For this review, take the finished solid that the model builds, in its own axes (mm). A direction names the side the tool comes from. Coordinates: 2 decimals unless noted, no trailing zeros. Loops run counter-clockwise (first coordinate to the right, second up) from the corner with the lowest first, then second, coordinate; pieces in that order, holes last.
```python
from build123d import *

# Parameters (mm, degrees)
SKETCH1_W           = 50
SKETCH1_H           = 60
BOSS_EXTRUDE1_DEPTH = 50
SKETCH2_W           = 30
SKETCH2_H           = 50
CUT_EXTRUDE1_DEPTH  = 77.811457479
SKETCH3_R           = 1.7
CUT_EXTRUDE2_DEPTH  = 64.442887702
SKETCH4_R           = 1.7
BOSS_EXTRUDE2_DEPTH = 50
CUT_EXTRUDE3_DEPTH  = 17
SKETCH7_W           = 10
SKETCH7_H           = 6
CUT_EXTRUDE4_DEPTH  = 10
SKETCH8_W           = 3
SKETCH8_H           = 17
CUT_EXTRUDE5_DEPTH  = 85.403791384
BOSS_EXTRUDE3_REACH = 61.363
SKETCH10_W          = 20
SKETCH10_H          = 12
SKETCH12_W          = 8
SKETCH12_H          = 16
CUT_EXTRUDE6_DEPTH  = 67.513156593


with BuildPart() as part:
    # Sketch1 → Boss-Extrude1 (new body)
    with BuildSketch(Plane.XY):
        Rectangle(SKETCH1_W, SKETCH1_H)
    extrude(amount=BOSS_EXTRUDE1_DEPTH)

    # Sketch2 → Cut-Extrude1 (cut, through all)
    with BuildSketch(Plane(origin=(25, 0, 0), x_dir=(0, 0, -1), z_dir=(1, 0, 0))):
        with Locations((-25, -5)):
            Rectangle(SKETCH2_W, SKETCH2_H)
    extrude(amount=-CUT_EXTRUDE1_DEPTH, mode=Mode.SUBTRACT)

    # Sketch3 → Cut-Extrude2 (cut, through all)
    with BuildSketch(Plane.XY.offset(50)):
        with Locations((-16.5, -24)):
            Circle(SKETCH3_R)
        with Locations((-16.5, 16)):
            Circle(SKETCH3_R)
        with Locations(Location((16.5, -24, 0), (0, 0, 90))):
            Circle(SKETCH3_R)
        with Locations(Location((16.5, 16, 0), (0, 0, 90))):
            Circle(SKETCH3_R)
    extrude(amount=-CUT_EXTRUDE2_DEPTH, mode=Mode.SUBTRACT)

    # Sketch4 → Boss-Extrude2 (add)
    # profile 1 of 2: a face of its own
    with BuildSketch(Plane.XY.offset(50)):
        with BuildLine():
            Line((-25, 30), (-25, 20))
            Line((-25, 20), (-27, 20))
            ThreePointArc((-27, 20), (-32, 25), (-27, 30))
            Line((-27, 30), (-25, 30))
        make_face()
        with Locations((-27, 25)):
            Circle(SKETCH4_R, mode=Mode.SUBTRACT)
    # profile 2 of 2: a face of its own
    with BuildSketch(Plane.XY.offset(50)):
        with BuildLine():
            Line((27, 30), (25, 30))
            Line((25, 30), (25, 20))
            Line((25, 20), (27, 20))
            ThreePointArc((27, 20), (32, 25), (27, 30))
        make_face()
        with Locations(Location((27, 25, 0), (0, 0, 180))):
            Circle(SKETCH4_R, mode=Mode.SUBTRACT)
    extrude(amount=-BOSS_EXTRUDE2_DEPTH)

    # Sketch6 → Cut-Extrude3 (cut)
    with BuildSketch(Plane.XY.offset(50)):
        with BuildLine():
            Line((25, 30), (25, 20))
            Line((25, 20), (27, 20))
            ThreePointArc((27, 20), (32, 25), (27, 30))
            Line((27, 30), (25, 30))
        make_face()
        with BuildLine():
            Line((-27, 30), (-25, 30))
            Line((-25, 30), (-25, 20))
            Line((-25, 20), (-27, 20))
            ThreePointArc((-27, 20), (-32, 25), (-27, 30))
        make_face()
    cut_extrude3 = extrude(amount=-CUT_EXTRUDE3_DEPTH, mode=Mode.SUBTRACT)

    # Sketch7 → Cut-Extrude4 (cut)
    with BuildSketch(Plane(origin=(0, 30, 0), x_dir=(1, 0, 0), z_dir=(0, 1, 0))):
        with Locations((27, -25)):
            Rectangle(SKETCH7_W, SKETCH7_H)
        with Locations((-27, -25)):
            Rectangle(SKETCH7_W, SKETCH7_H)
    extrude(amount=-CUT_EXTRUDE4_DEPTH, mode=Mode.SUBTRACT)

    # Mirror1: Cut-Extrude3 across plane
    add(cut_extrude3.mirror(Plane(origin=(0, 0, 25), x_dir=(1, 0, 0), z_dir=(0, 0, -1))), mode=Mode.SUBTRACT)

    # Sketch8 → Cut-Extrude5 (cut, through all)
    with BuildSketch(Plane(origin=(0, 30, 0), x_dir=(1, 0, 0), z_dir=(0, 1, 0))):
        with Locations((-23.5, -41.5)):
            Rectangle(SKETCH8_W, SKETCH8_H)
        with Locations((-23.5, -8.5)):
            Rectangle(SKETCH8_W, SKETCH8_H)
        with Locations((23.5, -41.5)):
            Rectangle(SKETCH8_W, SKETCH8_H)
        with Locations((23.5, -8.5)):
            Rectangle(SKETCH8_W, SKETCH8_H)
    extrude(amount=-CUT_EXTRUDE5_DEPTH, mode=Mode.SUBTRACT)

    # Sketch10 → Boss-Extrude3 (add, up to next)
    with BuildSketch(Plane.XY.offset(10), mode=Mode.PRIVATE) as boss_extrude3_sk1:
        with Locations((0, -24)):
            Rectangle(SKETCH10_W, SKETCH10_H)
    boss_extrude3_tool1 = extrude(boss_extrude3_sk1.sketch, amount=BOSS_EXTRUDE3_REACH, mode=Mode.PRIVATE) - part.part
    add(boss_extrude3_tool1.solids().sort_by_distance((0, -24, 10))[0])

    # Sketch12 → Cut-Extrude6 (cut, through all)
    with BuildSketch(Plane.XY.offset(50)):
        with Locations((-12, -5)):
            Rectangle(SKETCH12_W, SKETCH12_H)
        with Locations((12, -5)):
            Rectangle(SKETCH12_W, SKETCH12_H)
    extrude(amount=-CUT_EXTRUDE6_DEPTH, mode=Mode.SUBTRACT)


solid = part.part
```
Q1. Consider section B-B (y = -17). State the section outline as (x, z) points.
Q2. Consider section C-C (x = 11.5). State the section outline as (y, z) points.
Q3. The part is to be moulded in two halves that separate along Y. For faces 4 (the face through (17.15, -22.43, 45.07)), 5 (the face through (-22, 25, 25)), 6 (the face through (32, 25, 31)), say which applies: +Y half, -Y half, draft (parallel to the pull), parting line (faces both ways), or undercut.
Q4. Machinability: for faces 1 (the face through (22, 7, 44)), 2 (the face through (0, 20, 25)), 3 (the face through (-16, -5, 5)), which of the approach directions +Z, -Z, +X, -X, +Y, -Y give a long, thin tool a straight path to every point of the face, cutting with its end or side? Answer none if there is none.
Q5. For pin 1 Ø4 at (x, y) = (16.5, -24) entering from -Z; pin 2 Ø5 at (y, z) = (25.5, 25) entering from +X; pin 3 Ø3 at (y, z) = (-8, 4.5) entering from -X; pin 4 Ø2 at (x, y) = (-16.5, 16) entering from -Z, all flat-tipped, find the tip position at first contact; note any pin that passes through.
Q6. Wall thickness on probe 1 along Y at (x, z) = (-16.5, 47.75); probe 2 along Z at (x, y) = (25.5, 20.5); probe 3 along X at (y, z) = (17.5, 44): over which ranges is each line inside the solid? List them lowest first.
Q7. Consider section D-D (z = 45.5). State the section outline as (x, y) points.
Q8. Consider section A-A (z = 30). State the section outline as (x, y) points.
Model answer:
1. outline: (-22, 0) - (22, 0) - (22, 10) - (-22, 10) - close; (-22, 40) - (22, 40) - (22, 50) - (-22, 50) - close
2. outline: (-30, 0) - (-13, 0) - (-13, 10) - (-30, 10) - close; (-30, 40) - (-13, 40) - (-13, 50) - (-30, 50) - close; (3, 0) - (30, 0) - (30, 50) - (3, 50) - (3, 40) - (20, 40) - (20, 10) - (3, 10) - close
3. face 4: undercut
3. face 5: draft
3. face 6: parting line
4. face 1: +Z, +X, +Y, -Y
4. face 2: +X, -X
4. face 3: +Z, -Z
5. pin 1: stops at z = 0
5. pin 2: stops at x = 22
5. pin 3: stops at x = -22
5. pin 4: passes through
6. probe 1: y = -30 to -25.7, -22.3 to 14.3, 17.7 to 30
6. probe 2: z = 17 to 22, 28 to 33
6. probe 3: x = -22 to -17.3, -15.7 to 15.7, 17.3 to 22
7. outline: (-22, -30) - (22, -30) - (22, 30) - (-22, 30) - close; hole circle Ø3.4 at (-16.5, -24); hole circle Ø3.4 at (-16.5, 16); hole (-16, -13) - (-8, -13) - (-8, 3) - (-16, 3) - close; hole (8, -13) - (16, -13) - (16, 3) - (8, 3) - close; hole circle Ø3.4 at (16.5, -24); hole circle Ø3.4 at (16.5, 16)
8. outline: (-27, 20) - (27, 20) arc R5 ccw to (27, 30) - (-27, 30) arc R5 ccw to start; (-10, -30) - (10, -30) - (10, -18) - (-10, -18) - close; hole circle Ø3.4 at (-27, 25); hole circle Ø3.4 at (27, 25)
